```python
from build123d import *

# Parameters (mm, degrees)
SKETCH1_R           = 4.7625
BOSS_EXTRUDE1_DEPTH = 6.35


with BuildPart() as part:
    # Sketch1 → Boss-Extrude1 (new body)
    with BuildSketch(Plane.XY):
        with BuildLine():
            Line((-95.25, 50.8), (-95.25, 0))
            ThreePointArc((-95.25, 0), (-91.530256121, 8.980256121), (-82.55, 12.7))
            Line((-82.55, 12.7), (-69.85, 12.7))
            Line((-69.85, 12.7), (-69.85, 50.8))
            ThreePointArc((-69.85, 50.8), (-82.55, 63.5), (-95.25, 50.8))
        make_face()
        with Locations((-82.55, 50.8)):
            Circle(SKETCH1_R, mode=Mode.SUBTRACT)
        with BuildLine():
            ThreePointArc((-95.25, 0), (-91.530256121, -8.980256121), (-82.55, -12.7))
            ThreePointArc((-82.55, -12.7), (-73.569743879, -8.980256121), (-69.85, 0))
            Line((-69.85, 0), (-69.85, 12.7))
            Line((-69.85, 12.7), (-82.55, 12.7))
            ThreePointArc((-82.55, 12.7), (-91.530256121, 8.980256121), (-95.25, 0))
        make_face()
        with Locations((-82.55, 0)):
            Circle(SKETCH1_R, mode=Mode.SUBTRACT)
        with BuildLine():
            Line((-82.55, -12.7), (0, -12.7))
            ThreePointArc((0, -12.7), (12.7, 0), (0, 12.7))
            Line((0, 12.7), (-69.85, 12.7))
            Line((-69.85, 12.7), (-69.85, 0))
            ThreePointArc((-69.85, 0), (-73.569743879, -8.980256121), (-82.55, -12.7))
        make_face()
        Circle(SKETCH1_R, mode=Mode.SUBTRACT)
    extrude(amount=BOSS_EXTRUDE1_DEPTH)


solid = part.part
```
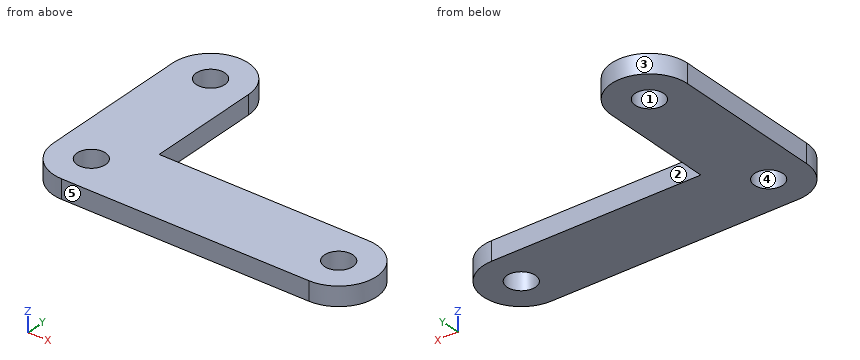
For this review, take the finished solid that the model builds, in its own axes (mm). Face numbers are marked on the shaded views. A direction names the side the tool comes from. Round coordinates to 2 decimals unless told otherwise and drop trailing zeros. Order: outer loops, then holes, each group sorted by start corner. A loop starts at its lowest first (then second) coordinate and runs counter-clockwise, first axis right, second up.
Q1. We need section A-A, the plane z = 4. State how many separate pieces and enclosed holes the cut face has, plus the area to 3 significant figures.
Findings below:
separate pieces: 1
enclosed holes: 3
area: 3,650 mm2
Q2. We need section D-D, the plane x = -58. Give the boundary of the cut face in (y, z), plus the area to 3 significant figures.
Findings below:
outline: (-12.7, 0) - (12.7, 0) - (12.7, 6.35) - (-12.7, 6.35) - close
area: 161 mm2
Q3. We need section B-B, the plane x = 1.5. Give the boundary of the cut face in (y, z).
Findings below:
outline: (-12.61, 0) - (-4.52, 0) - (-4.52, 6.35) - (-12.61, 6.35) - close; (4.52, 0) - (12.61, 0) - (12.61, 6.35) - (4.52, 6.35) - close
Q4. Wall thickness on line 1 (Y direction, x = -82.55, z = 4.5); line 2 (X direction, y = -4, z = 4.5); line 3 (Y direction, x = -69, z = 4.75): over which ranges is each line inside the solid? List them lowest first.
Findings below:
line 1: y = -12.7 to -4.76, 4.76 to 46.04, 55.56 to 63.5
line 2: x = -94.6 to -85.13, -79.97 to -2.58, 2.58 to 12.05
line 3: y = -12.7 to 12.7
Q5. Machinability: for the marked faces 1 and 2, which of the approach directions +Z, -Z, +X, -X, +Y, -Y give a long, thin tool a straight path to every point of the face, cutting with its end or side? Answer none if there is none.
Findings below:
face 1: +Z, -Z
face 2: +Z, -Z, +X, +Y
Q6. We need section C-C, the plane y = 21. Give the boundary of the cut face in (x, z), plus the area to 3 significant figures.
Findings below:
outline: (-95.25, 0) - (-69.85, 0) - (-69.85, 6.35) - (-95.25, 6.35) - close
area: 161 mm2
Q7. Mouldability with a two-part tool opening along X and no side actions: class the marked faces 3, 4 and 5 as pulls with the +X half, pulls with the -X half, needs draft (parallel to the pull), parting line crosses it, or undercut.
Findings below:
face 3: parting line crosses it
face 4: undercut
face 5: needs draft
